Work out the finished part from the listing and answer in its coordinate system (mm). A direction names the side the tool comes from. Coordinates: 2 decimals unless noted, no trailing zeros. Write each loop counter-clockwise with the first axis right and the second up, starting at its lowest first coordinate (ties: lowest second). Pieces come first, ordered by that corner, then holes. Notation, with made-up numbers: M 88.25,42 L 109.25,42 A14 cw 109.25,63 Z; hole C 25,57.5 d7. An arc over 180 degrees is marked long. Answer as CSV lines item,"result". Start each with the question number.
(1) A cutting plane is placed at D-D on y = 10. Give the vertices of the cut face in (x, z), then the cut area to 3 significant figures.
(2) A cutting plane is placed at A-A on z = 4.5. Give the vertices of the cut face in (x, y) (3 decimals), then the cut area to 3 significant figures.
(3) Find the intervals of material crossed by L1, parallel to Y at x = 7, z = -2; L2, parallel to Y at x = 13.5, z = -2.75; L3, parallel to X at y = -13, z = -6.5, in increasing order. Write a range as [from, to].
(4) A cutting plane is placed at B-B on x = -16. Give the vertices of the cut face in (y, z), then the cut area to 3 significant figures.
(5) Flat-ended cylindrical pins translate along their axes: P1, Ø12, axis at x = -13, z = -8, coming from the -Y side; P2, Ø3, axis at x = -16.5, z = 0.5, coming from the +Y side; P3, Ø5, axis at x = -0.5, z = -9, coming from the -Y side; P4, Ø5, axis at x = 13, y = -10, coming from the +Z side. Find the tip coordinate at first contact, or state that the pin passes through.
(6) The mould has two halves that part along X. Classify faces 3 (the cylindrical face through (-8.26, -8.16, 0.18)), 4 (the cylindrical face through (-5.506, -24.796, 0.178)), 5 (the flat face through (5, -5, -12.7)), 6 (the cylindrical face through (15.635, 15.795, 0.178)): released by +X, released by -X, zero draft, split by the parting line, or undercut.
(7) A cutting plane is placed at C-C on x = 2. Give the vertices of the cut face in (y, z), then the cut area to 3 significant figures.
(8) For faces 1 (the flat face through (5, -5, 12.7)), 2 (the flat face through (6.35, -16, 0)), determine the directions among +Z, -Z, +X, -X, +Y, -Y from which every point of the face is accessible in a straight line to the end or side of a thin tool.
from build123d import *

# Parameters (mm, degrees)
F0_R     = 25.4
F1_DEPTH = 12.7


with BuildPart() as f1:
    # F0 (on Top) → F1 (new body, symmetric)
    with BuildSketch(Plane.XY):
        Circle(F0_R)
        with BuildLine():
            ThreePointArc((-9.107237, -20.273353), (-15.715448, -15.715448), (-20.273353, -9.107237))
            ThreePointArc((-20.273353, -9.107237), (-20.13134, -7.243326), (-18.489298, -6.35))
            Line((-18.489298, -6.35), (-12.7, -6.35))
            ThreePointArc((-12.7, -6.35), (-8.209872, -8.209872), (-6.35, -12.7))
            Line((-6.35, -12.7), (-6.35, -18.489298))
            ThreePointArc((-6.35, -18.489298), (-7.243326, -20.13134), (-9.107237, -20.273353))
        make_face(mode=Mode.SUBTRACT)
        with BuildLine():
            ThreePointArc((0, 6.35), (4.490128, 4.490128), (6.35, 0))
            ThreePointArc((6.35, 0), (4.490128, -4.490128), (0, -6.35))
            ThreePointArc((0, -6.35), (-4.490128, -4.490128), (-6.35, 0))
            ThreePointArc((-6.35, 0), (-4.490128, 4.490128), (0, 6.35))
        make_face(mode=Mode.SUBTRACT)
        with BuildLine():
            Line((6.35, -18.489298), (6.35, -12.7))
            ThreePointArc((6.35, -12.7), (8.209872, -8.209872), (12.7, -6.35))
            Line((12.7, -6.35), (18.489298, -6.35))
            ThreePointArc((18.489298, -6.35), (20.13134, -7.243326), (20.273353, -9.107237))
            ThreePointArc((20.273353, -9.107237), (15.715448, -15.715448), (9.107237, -20.273353))
            ThreePointArc((9.107237, -20.273353), (7.243326, -20.13134), (6.35, -18.489298))
        make_face(mode=Mode.SUBTRACT)
        with BuildLine():
            Line((-6.35, 18.489298), (-6.35, 12.7))
            ThreePointArc((-6.35, 12.7), (-8.209872, 8.209872), (-12.7, 6.35))
            Line((-12.7, 6.35), (-18.489298, 6.35))
            ThreePointArc((-18.489298, 6.35), (-20.13134, 7.243326), (-20.273353, 9.107237))
            ThreePointArc((-20.273353, 9.107237), (-15.715448, 15.715448), (-9.107237, 20.273353))
            ThreePointArc((-9.107237, 20.273353), (-7.243326, 20.13134), (-6.35, 18.489298))
        make_face(mode=Mode.SUBTRACT)
        with BuildLine():
            ThreePointArc((12.7, 6.35), (8.209872, 8.209872), (6.35, 12.7))
            Line((6.35, 12.7), (6.35, 18.489298))
            ThreePointArc((6.35, 18.489298), (7.243326, 20.13134), (9.107237, 20.273353))
            ThreePointArc((9.107237, 20.273353), (15.715448, 15.715448), (20.273353, 9.107237))
            ThreePointArc((20.273353, 9.107237), (20.13134, 7.243326), (18.489298, 6.35))
            Line((18.489298, 6.35), (12.7, 6.35))
        make_face(mode=Mode.SUBTRACT)
    extrude(amount=F1_DEPTH, both=True)


solid = f1.part
Here are the results:
1,outline,"M -23.35,-12.7 L -19.85,-12.7 L -19.85,12.7 L -23.35,12.7 Z; M -6.95,-12.7 L 6.95,-12.7 L 6.95,12.7 L -6.95,12.7 Z; M 19.85,-12.7 L 23.35,-12.7 L 23.35,12.7 L 19.85,12.7 Z"
1,area,"531 mm^2"
2,outline,"C 0,0 d50.8; hole M -20.273,-9.107 A22.225 ccw -9.107,-20.273 A1.956 ccw -6.35,-18.489 L -6.35,-12.7 A6.35 ccw -12.7,-6.35 L -18.489,-6.35 A1.956 ccw Z; hole M -20.273,9.107 A1.956 ccw -18.489,6.35 L -12.7,6.35 A6.35 ccw -6.35,12.7 L -6.35,18.489 A1.956 ccw -9.107,20.273 A22.225 ccw Z; hole C 0,0 d12.7; hole M 6.35,-18.489 A1.956 ccw 9.107,-20.273 A22.225 ccw 20.273,-9.107 A1.956 ccw 18.489,-6.35 L 12.7,-6.35 A6.35 ccw 6.35,-12.7 Z; hole M 6.35,12.7 A6.35 ccw 12.7,6.35 L 18.489,6.35 A1.956 ccw 20.273,9.107 A22.225 ccw 9.107,20.273 A1.956 ccw 6.35,18.489 Z"
2,area,"1,350 mm^2"
3,L1,"y = [-24.42, -19.95], [-9.9, 9.9], [19.95, 24.42]"
3,L2,"y = [-21.52, -17.66], [-6.35, 6.35], [17.66, 21.52]"
3,L3,"x = [-21.82, -18.03], [-6.35, 6.35], [18.03, 21.82]"
4,outline,"M -19.73,-12.7 L -15.43,-12.7 L -15.43,12.7 L -19.73,12.7 Z; M -6.35,-12.7 L 6.35,-12.7 L 6.35,12.7 L -6.35,12.7 Z; M 15.43,-12.7 L 19.73,-12.7 L 19.73,12.7 L 15.43,12.7 Z"
4,area,"541 mm^2"
5,P1,"stops at y = -24.42"
5,P2,"stops at y = 20.5"
5,P3,"stops at y = -25.4"
5,P4,"passes through"
6,face 3,"undercut"
6,face 4,"split by the parting line"
6,face 5,"zero draft"
6,face 6,"undercut"
7,outline,"M -25.32,-12.7 L -6.03,-12.7 L -6.03,12.7 L -25.32,12.7 Z; M 6.03,-12.7 L 25.32,-12.7 L 25.32,12.7 L 6.03,12.7 Z"
7,area,"980 mm^2"
8,face 1,"+Z, +X, -X, +Y, -Y"
8,face 2,"+Z, -Z"
